The model under review builds one solid part; all positions refer to its coordinate system, in mm. A direction names the side the tool comes from. Round coordinates to 2 decimals unless told otherwise and drop trailing zeros. Write each loop counter-clockwise with the first axis right and the second up, starting at its lowest first coordinate (ties: lowest second). Pieces come first, ordered by that corner, then holes. Notation, with made-up numbers: (7.25, 25.25) -> (64.25, 25.25) arc R24 cw to (64.25, 46.25) -> close; hole circle Ø6 at (-30, 22.5). An arc over 180 degrees is marked (long way). Answer as a JSON object with one key per item and string values. Group by question number.
1) Mouldability with a two-part tool opening along Z and no side actions: class faces 5 (the flat face through (9.4, 2.5, 10.3)), 6 (the flat face through (1.8, 4.5, 0.5)), 7 (the flat face through (15.3, 6, 5)), 8 (the cylindrical face through (10.886, 4.36, 5.192)) as pulls with the +Z half, pulls with the -Z half, needs draft (parallel to the pull), parting line crosses it, or undercut.
2) Insertion check: pin 1 Ø2.5 at (x, z) = (1, 3) entering from +Y; pin 2 Ø5 at (x, y) = (11.5, 5) entering from +Z; pin 3 Ø4.5 at (x, y) = (8.5, 4.5) entering from -Z; pin 4 Ø3.5 at (x, z) = (9.3, 5.4) entering from +Y. Each pin has a flat end and moves straight along its axis. Give the tip position at first contact, or say it passes through.
3) We need section A-A, the plane y = 6.75. Count the separate pieces of the cut face and the enclosed holes in it, then the cut area to 3 significant figures.
4) Machinability: for faces 1 (the flat face through (9.4, 3.7, 1)), 2 (the flat face through (1.8, 4.5, 10.3)), 3 (the flat face through (2, 7, 5)), 4 (the cylindrical face through (11.1, 6.3, 7.8)), which of the approach directions +Z, -Z, +X, -X, +Y, -Y give a long, thin tool a straight path to every point of the face, cutting with its end or side? Answer none if there is none.
5) We need section C-C, the plane z = 5.4. Write out the cut boundary in (x, y).
6) We need section D-D, the plane y = 1.25. Write out the cut boundary in (x, z), then the cut area to 3 significant figures.
7) To check wall thickness, follow probe 1 along X at (y, z) = (5.25, 5.4); probe 2 along X at (y, z) = (5.5, 1.75); probe 3 along X at (y, z) = (3.75, 5.4). State the ranges of each line that lie inside material, in increasing order. Write a range as [from, to].
from build123d import *

# Parameters (mm, degrees)
BOSS_EXTRUDE1_DEPTH      = 10.8
SKETCH2_R                = 3
BOSS_EXTRUDE2_DEPTH      = 4.6
SKETCH3_R                = 1.6
CUT_EXTRUDE1_DEPTH       = 24.163764806
CHAMFER1_SIZE            = 1
SKETCH4_W                = 16
SKETCH4_H                = 5
CUT_EXTRUDE2_DEPTH       = 1
CHAMFER2_SIZE            = 1
CHAMFER2_OF_MIRROR1_SIZE = 1


with BuildPart() as part:
    # Sketch1 → Boss-Extrude1 (new body)
    with BuildSketch(Plane.XY):
        Polygon((0, 0), (18.6, 0), (18.6, 7), (15.3, 7), (15.3, 4), (3.3, 4), (3.3, 7), (0, 7), align=None)
    extrude(amount=BOSS_EXTRUDE1_DEPTH)

    # Sketch2 → Boss-Extrude2 (add)
    with BuildSketch(Plane(origin=(0, 4, 0), x_dir=(1, 0, 0), z_dir=(0, 1, 0))):
        with Locations(Location((9.3, -5.4, 0), (0, 0, 90))):
            Circle(SKETCH2_R)
    extrude(amount=BOSS_EXTRUDE2_DEPTH)

    # Sketch3 → Cut-Extrude1 (cut, through all)
    with BuildSketch(Plane(origin=(0, 8.6, 0), x_dir=(1, 0, 0), z_dir=(0, 1, 0))):
        with Locations(Location((9.3, -5.4, 0), (0, 0, 270))):
            Circle(SKETCH3_R)
    extrude(amount=-CUT_EXTRUDE1_DEPTH, mode=Mode.SUBTRACT)

    # Chamfer1
    chamfer1_edges = [part.edges().sort_by_distance(p)[0] for p in [
        (18.6, 0, 5.4),
        (0, 0, 5.4),
    ]]
    chamfer(chamfer1_edges, length=CHAMFER1_SIZE)

    # Sketch4 → Cut-Extrude2 (cut)
    with BuildSketch(Plane(origin=(0, 0, 0), x_dir=(-1, 0, 0), z_dir=(0, 0, -1))):
        with Locations((-9.3, 4.5)):
            Rectangle(SKETCH4_W, SKETCH4_H)
    cut_extrude2 = extrude(amount=-CUT_EXTRUDE2_DEPTH, mode=Mode.SUBTRACT)

    # Chamfer2
    chamfer2_edges = [part.edges().sort_by_distance(p)[0] for p in [
        (1.3, 4.5, 1),
        (17.3, 4.5, 1),
        (9.3, 2, 1),
    ]]
    chamfer(chamfer2_edges, length=CHAMFER2_SIZE - 0.0001)  # a hair under: the kernel refuses the full size

    # Mirror1: Cut-Extrude2 across plane
    add(cut_extrude2.mirror(Plane(origin=(0, 0, 5.4), x_dir=(1, 0, 0), z_dir=(0, 0, -1))), mode=Mode.SUBTRACT)

    # Chamfer2 of Mirror1
    chamfer2_of_mirror1_edges = [part.edges().sort_by_distance(p)[0] for p in [
        (1.3, 4.5, 9.8),
        (17.3, 4.5, 9.8),
        (9.3, 2, 9.8),
    ]]
    chamfer(chamfer2_of_mirror1_edges, length=CHAMFER2_OF_MIRROR1_SIZE - 0.0001)  # a hair under: the kernel refuses the full size


solid = part.part
Here are the results:
{
 "1": {"face 5": "pulls with the +Z half", "face 6": "pulls with the -Z half", "face 7": "needs draft", "face 8": "undercut"},
 "2": {"pin 1": "stops at y = 7", "pin 2": "stops at z = 10.3", "pin 3": "stops at z = 0.25", "pin 4": "stops at y = 8.6"},
 "3": {"separate pieces": "3", "enclosed holes": "1", "area": "85.5 mm^2"},
 "4": {"face 1": "-Z, +Y", "face 2": "+Z, +Y", "face 3": "+Z, -Z, -X, +Y", "face 4": "+Y"},
 "5": {"outline": "(0, 1) -> (1, 0) -> (7.7, 0) -> (7.7, 8.6) -> (6.3, 8.6) -> (6.3, 4) -> (3.3, 4) -> (3.3, 7) -> (0, 7) -> close; (10.9, 0) -> (17.6, 0) -> (18.6, 1) -> (18.6, 7) -> (15.3, 7) -> (15.3, 4) -> (12.3, 4) -> (12.3, 8.6) -> (10.9, 8.6) -> close"},
 "6": {"outline": "(0, 0) -> (18.6, 0) -> (18.6, 10.8) -> (0, 10.8) -> close; hole circle Ø3.2 at (9.3, 5.4)", "area": "193 mm^2"},
 "7": {"probe 1": "x = [0, 3.3], [6.3, 7.7], [10.9, 12.3], [15.3, 18.6]", "probe 2": "x = [0, 3.3], [15.3, 18.6]", "probe 3": "x = [0, 7.7], [10.9, 18.6]"}
}
